The figure shows three views and two pictorial views of one solid part (mm, origin at its lowest corner). Answer the questions. A direction names the side the tool comes from. Coordinates: 2 decimals unless noted, no trailing zeros. Order: outer loops, then holes, each group sorted by start corner. A loop starts at its lowest first (then second) coordinate and runs counter-clockwise, first axis right, second up. Notation, with made-up numbers: (10, -29) -> (62, -29) arc R20 ccw to (62, 1) -> close; hole circle Ø4 at (16, 61). An arc over 180 degrees is marked (long way). Write item = value, one per line. Start each with the question number.
Q1. For a pull along Z with two mould halves and no side action, classify the marked faces 1, 2 and 3 as +Z half, -Z half, draft (parallel to the pull), parting line (faces both ways), or undercut.
Q2. Straight lines are drawn through the part: L1, parallel to X at y = 8.5, z = 2.5; L2, parallel to Z at x = 28, y = 9.25; L3, parallel to Y at x = 24.5, z = 1. For each, find the intervals that lie inside material, in ascending order. Write a range as from..to.
Q3. Flat-ended cylindrical pins translate along their axes: pin 1 (2.5 mm diameter, centred on x = 35.5, z = 1.5, fed in from +Y); pin 2 (0.6 mm diameter, centred on x = 114, y = 10.5, fed in from +Z). Find the tip coordinate at first contact, or state that the pin passes through.
Q4. The part is cut by section A-A, the plane x = 34.5. Determine the outline of the cut face in (y, z), plus the area to 3 significant figures.
Q5. The part is cut by section C-C, the plane z = 7.25. Determine the outline of the cut face in (x, y), plus the area to 3 significant figures.
Q6. The part is cut by section B-B, the plane y = 1.25. Determine the outline of the cut face in (x, z), plus the area to 3 significant figures.
Q7. Which of the six approach directions +Z, -Z, +X, -X, +Y, -Y give full straight-line access (tool end or side, diameter ignored) to the marked faces 4 and 5?
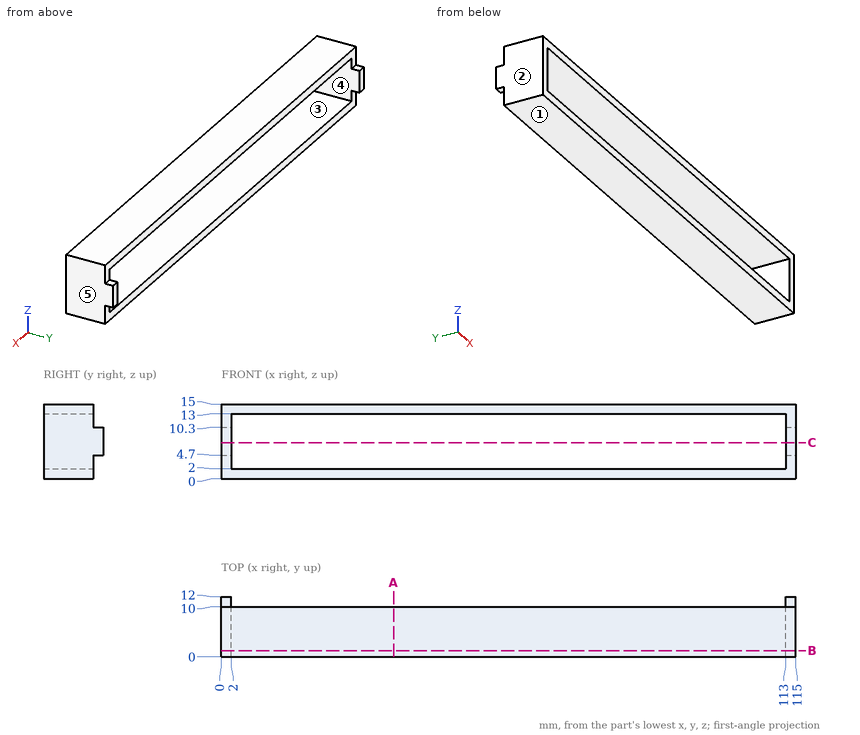
Model answer:
q1.face_1 = -Z half
q1.face_2 = draft
q1.face_3 = undercut
q2.L1 = 0..2, 113..115
q2.L2 = 0..2, 13..15
q2.L3 = 0..10
q3.pin_1 = 10
q3.pin_2 = 10.3
q4.outline = (0, 0) -> (10, 0) -> (10, 2) -> (0, 2) -> close; (0, 13) -> (10, 13) -> (10, 15) -> (0, 15) -> close
q4.area = 40.0 mm2
q5.outline = (0, 0) -> (2, 0) -> (2, 12) -> (0, 12) -> close; (113, 0) -> (115, 0) -> (115, 12) -> (113, 12) -> close
q5.area = 48.0 mm2
q6.outline = (0, 0) -> (115, 0) -> (115, 15) -> (0, 15) -> close; hole (2, 2) -> (113, 2) -> (113, 13) -> (2, 13) -> close
q6.area = 504 mm2
q7.face_4 = +Y, -Y
q7.face_5 = +Z, -Z, +X, +Y, -Y
